```python
from build123d import *

# Parameters (mm, degrees)
SKETCH1_W          = 37.5
SKETCH1_H          = 110
CUT_EXTRUDE2_DEPTH = 100
CUT_EXTRUDE3_DEPTH = 139.315761936


with BuildPart() as part:
    # Sketch1 → Revolve3 (revolve)
    with BuildSketch(Plane.XY, mode=Mode.PRIVATE) as revolve3_sk:
        with Locations((18.75, 55)):
            Rectangle(SKETCH1_W, SKETCH1_H)
    revolve(revolve3_sk.sketch.rotate(Axis((37.5, 0, 0), (0, 1, 0)), 270), axis=Axis((37.5, 0, 0), (0, 1, 0)))

    # Sketch2 → Cut-Extrude2 (cut)
    with BuildSketch(Plane(origin=(0, 0, 0), x_dir=(-1, 0, 0), z_dir=(0, -1, 0))):
        with BuildLine():
            ThreePointArc((-2.5, 0), (-37.5, 35), (-72.5, 0))
            Line((-72.5, 0), (-2.5, 0))
        make_face()
        with BuildLine():
            Line((-2.5, 0), (-72.5, 0))
            ThreePointArc((-72.5, 0), (-37.5, -35), (-2.5, 0))
        make_face()
    extrude(amount=-CUT_EXTRUDE2_DEPTH, mode=Mode.SUBTRACT)

    # Sketch3 → Cut-Extrude3 (cut, through all)
    with BuildSketch(Plane(origin=(0, 110, 0), x_dir=(1, 0, 0), z_dir=(0, 1, 0))):
        with BuildLine():
            ThreePointArc((49.5, 0), (37.5, 12), (25.5, 0))
            Line((25.5, 0), (49.5, 0))
        make_face()
        with BuildLine():
            Line((49.5, 0), (25.5, 0))
            ThreePointArc((25.5, 0), (37.5, -12), (49.5, 0))
        make_face()
    extrude(amount=-CUT_EXTRUDE3_DEPTH, mode=Mode.SUBTRACT)


solid = part.part
```
Here's how the part is built. I have some questions about the finished solid (model axes, mm). A direction names the side the tool comes from. Round coordinates to 2 decimals unless told otherwise and drop trailing zeros. Write each loop counter-clockwise with the first axis right and the second up, starting at its lowest first coordinate (ties: lowest second). Pieces come first, ordered by that corner, then holes. Notation, with made-up numbers: M 89,52.5 L 115,52.5 A16 cw 115,58.5 Z; hole C 81,58 d3. An arc over 180 degrees is marked long. Answer as CSV lines item,"result". Start each with the question number.
1. Suppose I cut it at A-A on x = 37.5. Write out the boundary of the cut face in (y, z).
2. Suppose I cut it at D-D on z = -21. Write out the boundary of the cut face in (x, y), then the cut area to 3 significant figures.
3. Suppose I cut it at B-B on z = 0. Write out the boundary of the cut face in (x, y).
4. On a 3-axis mill with a long thin cutter (end or side, diameter ignored), from which of +Z, -Z, +X, -X, +Y, -Y can I reach the whole of each face in a straight line? I mean faces 1 (the flat face through (22, 100, 0)), 2 (the cylindrical face through (49.49, 105.07, 0.53)). Say none if no direction works.
5. Suppose I cut it at C-C on y = 30.5. Write out the boundary of the cut face in (x, z), then the cut area to 3 significant figures.
6. Thinking about a two-plate mould opening in X: for faces 3 (the cylindrical face through (60, 56, 30)), 4 (the flat face through (71, 0, 11)), 5 (the cylindrical face through (9.73, 49.3, -21.3)), which applies, released by +X, released by -X, zero draft, split by the parting line, or undercut?
7. I'm going to push flat-ended pins straight in: pin 1 Ø6 at (x, z) = (65.5, -20.5) entering from -Y; pin 2 Ø12 at (y, z) = (51, -18.5) entering from -X; pin 3 Ø6 at (x, y) = (50, 47.5) entering from -Z; pin 4 Ø2 at (y, z) = (62, 16) entering from -X. Where does each tip first touch, or does it pass through?
8. I need wall thicknesses on probe 1 along Z at (x, y) = (37, 106); probe 2 along Y at (x, z) = (52.5, -3.5); probe 3 along Z at (x, y) = (29, 6). Which ranges of each line are inside material? Lowest first, please.
Check result:
1,outline,"M 0,-37.5 L 110,-37.5 L 110,-12 L 100,-12 L 100,-35 L 0,-35 Z; M 0,35 L 100,35 L 100,12 L 110,12 L 110,37.5 L 0,37.5 Z"
2,outline,"M 6.43,0 L 9.5,0 L 9.5,100 L 65.5,100 L 65.5,0 L 68.57,0 L 68.57,110 L 6.43,110 Z"
2,area,"1,240 mm2"
3,outline,"M 0,0 L 2.5,0 L 2.5,100 L 25.5,100 L 25.5,110 L 0,110 Z; M 49.5,100 L 72.5,100 L 72.5,0 L 75,0 L 75,110 L 49.5,110 Z"
4,face 1,"-Y"
4,face 2,"+Y, -Y"
5,outline,"C 37.5,0 d75; hole C 37.5,0 d70"
5,area,"569 mm2"
6,face 3,"split by the parting line"
6,face 4,"zero draft"
6,face 5,"undercut"
7,pin 1,"stops at y = 0"
7,pin 2,"stops at x = 2.14"
7,pin 3,"stops at z = -36.28"
7,pin 4,"stops at x = 3.13"
8,probe 1,"z = -37.5 to -11.99, 11.99 to 37.5"
8,probe 2,"y = 100 to 110"
8,probe 3,"z = -36.52 to -33.95, 33.95 to 36.52"
